Source: three-view drawing plus pictorial views. Frame: mm from the lowest corner of the part. A direction names the side the tool comes from. Give positions to 0.01 mm unless a question says otherwise; leave off trailing zeros. Loops run counter-clockwise (first coordinate to the right, second up) from the corner with the lowest first, then second, coordinate; pieces in that order, holes last. Notation, with made-up numbers: M 18,-29.5 L 70,-29.5 A29 ccw 70,-8.5 Z; hole C 86.5,-9.5 d6. An arc over 180 degrees is marked long. One line per item, written item: value. Start each with the question number.
(1) Access query for the marked faces 4, 5 and 6. Directions: +Z, -Z, +X, -X, +Y, -Y. A direction counts if a zero-diameter tool reaches every point of the face in a straight line with its end or side. Return the directions, or none.
(2) Section B-B on y = 63.5. Output: boundary loops of the cut face in (x, z), plus the area to 3 significant figures.
(3) Section A-A on x = 63.5. Output: boundary loops of the cut face in (y, z).
(4) Section D-D on y = 91. Output: boundary loops of the cut face in (x, z), plus the area to 3 significant figures.
(5) Section C-C on z = 87. Output: boundary loops of the cut face in (x, y).
(6) Ray query, line 1 along X through (y, z) = (63, 39); line 2 along Z through (x, y) = (85.5, 117). Return the intervals inside material, ascending. Write a range as from..to.
(7) Pull-direction query (Y, two-part tool) for the marked faces 1, 2 and 3; classes: released by +Y, released by -Y, zero draft, split by the parting line, or undercut.
(8) Pin query (flat end, axial travel): P1, Ø20.5, axis at x = 52.5, z = 94.5, coming from the +Y side; P2, Ø10, axis at y = 71.5, z = 23, coming from the +X side; P3, Ø4, axis at x = 67, z = 29, coming from the -Y side. Return the tip coordinate at first contact, or that it passes through.
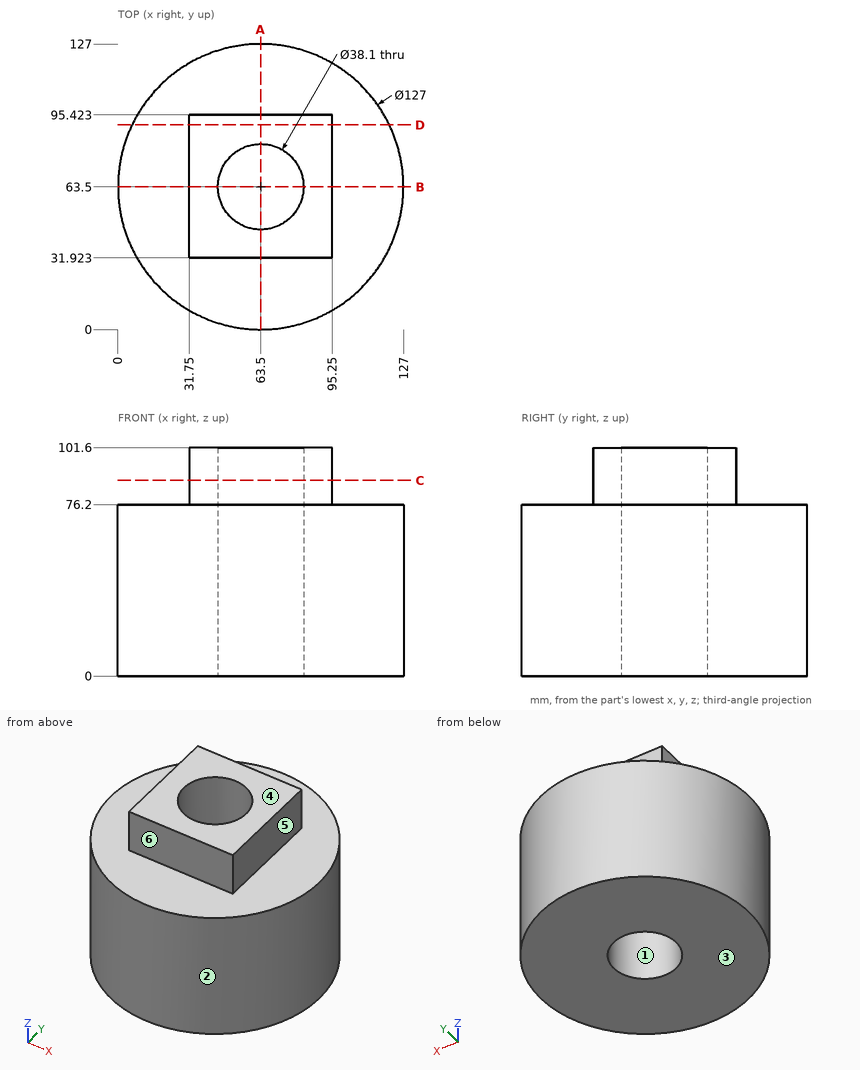
Output values:
1. face 4: +Z, +X, -X, +Y, -Y
1. face 5: +Z, +X, +Y, -Y
1. face 6: +Z, +X, -X, -Y
2. outline: M 0,0 L 44.45,0 L 44.45,101.6 L 31.75,101.6 L 31.75,76.2 L 0,76.2 Z; M 82.55,0 L 127,0 L 127,76.2 L 95.25,76.2 L 95.25,101.6 L 82.55,101.6 Z
2. area: 7,420 mm²
3. outline: M 0,0 L 44.45,0 L 44.45,101.6 L 31.92,101.6 L 31.92,76.2 L 0,76.2 Z; M 82.55,0 L 127,0 L 127,76.2 L 95.42,76.2 L 95.42,101.6 L 82.55,101.6 Z
4. outline: M 6.26,0 L 120.74,0 L 120.74,76.2 L 95.25,76.2 L 95.25,101.6 L 31.75,101.6 L 31.75,76.2 L 6.26,76.2 Z
4. area: 10,300 mm²
5. outline: M 31.75,31.92 L 95.25,31.92 L 95.25,95.42 L 31.75,95.42 Z; hole C 63.5,63.5 d38.1
6. line 1: x = 0..44.46, 82.54..127
6. line 2: z = 0..76.2
7. face 1: undercut
7. face 2: split by the parting line
7. face 3: zero draft
8. P1: stops at y = 95.42
8. P2: stops at x = 126.93
8. P3: stops at y = 0.02
